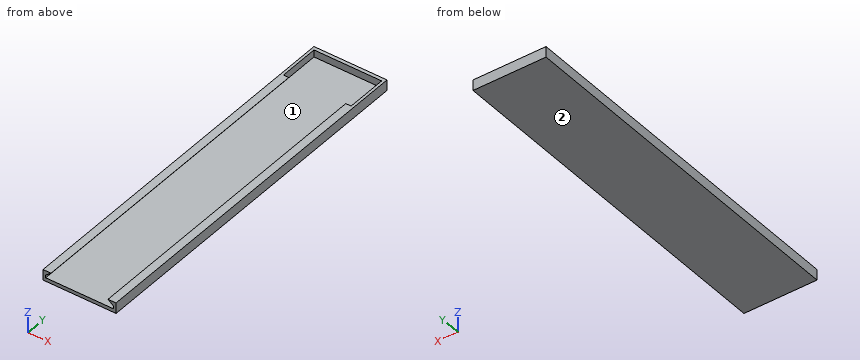
from build123d import *

# Parameters (mm, degrees)
F1_DEPTH = 202
F2_W     = 41
F2_H     = 6
F3_DEPTH = 2
F5_W     = 38
F5_H     = 23
F6_DEPTH = 4


with BuildPart() as f1:
    # F0 (on Front) → F1 (new body)
    with BuildSketch(Plane.XZ):
        Polygon((-20.5, 6), (-20.5, 0), (20.5, 0), (20.5, 6), (16, 6), (19, 3.6), (19, 2), (-19, 2), (-19, 3.6), (-16, 6), align=None)
    extrude(amount=F1_DEPTH)

    # F2 (on Front) → F3 (join)
    with BuildSketch(Plane.XZ):
        with Locations((0, 3)):
            Rectangle(F2_W, F2_H)
    extrude(amount=-F3_DEPTH)

    # F5 (on offset) → F6 (cut)
    with BuildSketch(Plane.XY.offset(6)):
        with Locations((0, -11.5)):
            Rectangle(F5_W, F5_H)
    extrude(amount=-F6_DEPTH, mode=Mode.SUBTRACT)


solid = f1.part
The listing builds one solid part. Answer for the finished solid, in the listing's coordinates (mm). Face numbers are marked on the shaded views. Give positions to 0.01 mm unless a question says otherwise; leave off trailing zeros. Order: outer loops, then holes, each group sorted by start corner. A loop starts at its lowest first (then second) coordinate and runs counter-clockwise, first axis right, second up. Notation, with made-up numbers: (11.25, 66) - (19.25, 66) arc R26 cw to (19.25, 90) - close; hole circle Ø4 at (59, 66). An arc over 180 degrees is marked (long way). Use one line per item in the form item = value.
1) Find section A-A on y = -184. Determine the outline of the cut face in (x, z).
Verdict:
outline = (-20.5, 0) - (20.5, 0) - (20.5, 6) - (16, 6) - (19, 3.6) - (19, 2) - (-19, 2) - (-19, 3.6) - (-16, 6) - (-20.5, 6) - close
2) Find section B-B on x = -7.5. Determine the outline of the cut face in (y, z).
Verdict:
outline = (-202, 0) - (2, 0) - (2, 6) - (0, 6) - (0, 2) - (-202, 2) - close
3) Each of these flat-tipped pins is pushed along its axis until it touches: pin 1 (2 mm diameter, centred on x = 13, z = 4, fed in from -Y); pin 2 (2 mm diameter, centred on x = 4.5, y = -173.5, fed in from +Z). Where does it stop, or does it pass through?
Verdict:
pin_1 = 0
pin_2 = 2
4) Consider probe 1 along X at (y, z) = (-187, 2.4); probe 2 along Y at (x, z) = (-17.5, 4.95); probe 3 along Z at (x, y) = (-14, -28). Determine where each line is inside the solid, lowest interval first. Write a range as [from, to].
Verdict:
probe_1 = [-20.5, -19], [19, 20.5]
probe_2 = [-202, -23], [0, 2]
probe_3 = [0, 2]
5) The mould has two halves that part along X. Classify the marked faces 1 and 2: released by +X, released by -X, zero draft, split by the parting line, or undercut.
Verdict:
face_1 = undercut
face_2 = zero draft
